Part print with two shaded views. Sizes in mm from the minimum x, y, z corner. Coordinates: 2 decimals unless noted, no trailing zeros. Write each loop counter-clockwise with the first axis right and the second up, starting at its lowest first coordinate (ties: lowest second). Pieces come first, ordered by that corner, then holes.
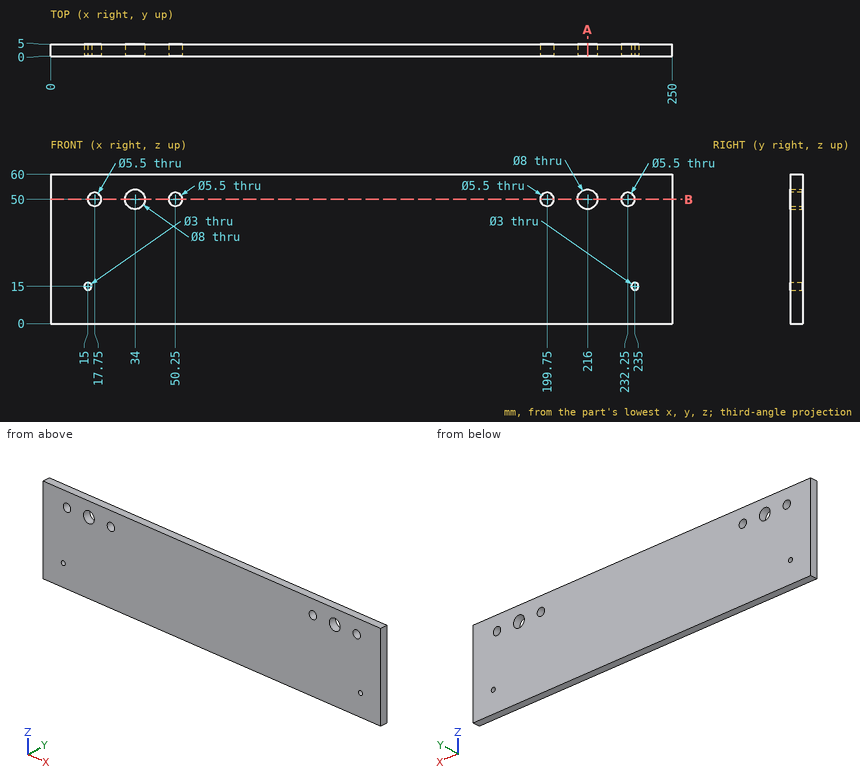
(1) Probe L1, parallel to X at y = 3, z = 15; L2, parallel to Z at x = 216, y = 2.35; L3, parallel to Z at x = 17.75, y = 3.6. List the from-to ranges inside material, lowest first.
(2) Flat gauge pins, fed straight in: P1, Ø9, axis at x = 232.25, z = 50, coming from the -Y side; P2, Ø5, axis at x = 50.25, z = 50, coming from the -Y side. Where does each tip first touch, or does it go through?
(3) Slice it at A-A, the plane x = 216. List the corners of the cut face in (y, z), and give its area (3 significant figures).
(4) Slice it at B-B, the plane z = 50. List the corners of the cut face in (x, y), and give its area (3 significant figures).
Results:
1. L1: x = 0 to 13.5, 16.5 to 233.5, 236.5 to 250
1. L2: z = 0 to 46, 54 to 60
1. L3: z = 0 to 47.25, 52.75 to 60
2. P1: stops at y = 0
2. P2: passes through
3. outline: (0, 0) - (5, 0) - (5, 46) - (0, 46) - close; (0, 54) - (5, 54) - (5, 60) - (0, 60) - close
3. area: 260 mm2
4. outline: (0, 0) - (15, 0) - (15, 5) - (0, 5) - close; (20.5, 0) - (30, 0) - (30, 5) - (20.5, 5) - close; (38, 0) - (47.5, 0) - (47.5, 5) - (38, 5) - close; (53, 0) - (197, 0) - (197, 5) - (53, 5) - close; (202.5, 0) - (212, 0) - (212, 5) - (202.5, 5) - close; (220, 0) - (229.5, 0) - (229.5, 5) - (220, 5) - close; (235, 0) - (250, 0) - (250, 5) - (235, 5) - close
4. area: 1,060 mm2
